from build123d import *

# Parameters (mm, degrees)
SKETCH2_W           = 134.477697302
SKETCH2_H           = 109.076354478
BOSS_EXTRUDE1_DEPTH = 84.074
SKETCH3_R           = 12.7
CUT_EXTRUDE1_DEPTH  = 127
SKETCH4_W           = 81.978128355
SKETCH4_H           = 50.707128689
CUT_EXTRUDE2_DEPTH  = 104.14
BOSS_EXTRUDE2_DEPTH = 25.4
BOSS_EXTRUDE3_DEPTH = 25.4


with BuildPart() as part:
    # Sketch2 → Boss-Extrude1 (new body)
    with BuildSketch(Plane.XY):
        Rectangle(SKETCH2_W, SKETCH2_H)
    extrude(amount=BOSS_EXTRUDE1_DEPTH)

    # Sketch3 → Cut-Extrude1 (cut)
    with BuildSketch(Plane.XY.offset(84.074)):
        Circle(SKETCH3_R)
    extrude(amount=-CUT_EXTRUDE1_DEPTH, mode=Mode.SUBTRACT)

    # Sketch4 → Cut-Extrude2 (cut)
    with BuildSketch(Plane(origin=(0, 54.538177239, 0), x_dir=(1, 0, 0), z_dir=(0, 1, 0))):
        with Locations((-7.023947617, -26.021677284)):
            Rectangle(SKETCH4_W, SKETCH4_H)
    extrude(amount=-CUT_EXTRUDE2_DEPTH, mode=Mode.SUBTRACT)

    # Sketch5 → Boss-Extrude2 (add)
    with BuildSketch(Plane(origin=(67.238848651, 0, 0), x_dir=(0, 0, -1), z_dir=(1, 0, 0))):
        Polygon((-54.326321663, 1.325818935), (-44.711130396, 12.412030691), (-49.504475775, 26.282136468), (-63.913012421, 29.06603049), (-73.528203689, 17.979818734), (-68.734858309, 4.109712956), align=None)
    extrude(amount=BOSS_EXTRUDE2_DEPTH)

    # Sketch6 → Boss-Extrude3 (add)
    with BuildSketch(Plane(origin=(67.238848651, 0, 0), x_dir=(0, 0, -1), z_dir=(1, 0, 0))):
        Polygon((-33.317190853, -32.329584791), (-34.779908073, -16.333922758), (-49.363916354, -9.602842013), (-62.485207415, -18.867423301), (-61.022490195, -34.863085333), (-46.438481914, -41.594166078), align=None)
    extrude(amount=BOSS_EXTRUDE3_DEPTH)


solid = part.part
Geometry: final body of the model. Coordinates: model frame, mm. A direction names the side the tool comes from. Round coordinates to 2 decimals unless told otherwise and drop trailing zeros. Order: outer loops, then holes, each group sorted by start corner. A loop starts at its lowest first (then second) coordinate and runs counter-clockwise, first axis right, second up. Notation, with made-up numbers: (31, -37.75) -> (78, -37.75) arc R15 ccw to (78, -22.75) -> close; hole circle Ø4 at (-34.5, -5.75). An arc over 180 degrees is marked (long way). Put each result on its own line as item: value. Start each with the question number.
Q1. Section A-A on x = 0. Return the cut outline in (y, z), and give its area (3 significant figures).
Q2. Line query: probe 1 along Y at (x, z) = (0, 58.5); probe 2 along Z at (x, y) = (33.5, 22.5); probe 3 along X at (y, z) = (-38, 43.5). Output: solid intervals per line, ascending.
Q3. Reachability of faces 1 (the flat face through (79.761, 23.601, 68.653)), 2 (the flat face through (79.761, -26.753, 61.764)), 3 (the flat face through (79.761, -37.027, 39.97)), 4 (the flat face through (79.761, 19.25, 47.074)), 5 (the flat face through (79.761, 6.791, 49.586)) from +Z, -Z, +X, -X, +Y, -Y: full face, straight path, thin tool, end or side. Return the list, or none.
Q4. Pull-direction query (Y, two-part tool) for faces 6 (the flat face through (-1, 54.538, 60)), 7 (the flat face through (-67.239, -1, 41)), 8 (the flat face through (79.761, 2.737, 61.631)), 9 (the cylindrical face through (-2.75, -12.4, 0.34)); classes: +Y half, -Y half, draft (parallel to the pull), parting line (faces both ways), or undercut.
Q5. Section B-B on y = -5. Return the cut outline in (x, z).
Q6. Section C-C on z = 31. Return the cut outline in (x, y), and give its area (3 significant figures).
Q7. Section D-D on y = -39.5. Return the cut outline in (x, z), and give its area (3 significant figures).
Q8. First-contact query: pin 1 (12 mm diameter, centred on y = -43, z = 35.5, fed in from +X); pin 2 (12 mm diameter, centred on x = 55, y = -25.5, fed in from -Z); pin 3 (12 mm diameter, centred on x = -6.5, z = 23.5, fed in from +Y); pin 4 (4 mm diameter, centred on x = 72.5, y = 26, fed in from +Z). Flat tips, straight axial feed; report the tip coordinate or a pass-through.
Ans:
1. outline: (-54.54, 0) -> (-12.7, 0) -> (-12.7, 0.67) -> (-49.6, 0.67) -> (-49.6, 51.38) -> (-12.7, 51.38) -> (-12.7, 84.07) -> (-54.54, 84.07) -> close; (12.7, 0) -> (54.54, 0) -> (54.54, 0.67) -> (12.7, 0.67) -> close; (12.7, 51.38) -> (54.54, 51.38) -> (54.54, 84.07) -> (12.7, 84.07) -> close
1. area: 3,040 mm2
2. probe 1: y = -54.54 to -12.7, 12.7 to 54.54
2. probe 2: z = 0 to 0.67, 51.38 to 84.07
2. probe 3: x = -67.24 to -48.01, 33.97 to 92.64
3. face 1: +Z, +X, +Y
3. face 2: +Z, +X, -Y
3. face 3: -Z, +X, -Y
3. face 4: -Z, +X, +Y
3. face 5: -Z, +X
4. face 6: +Y half
4. face 7: draft
4. face 8: undercut
4. face 9: undercut
5. outline: (-67.24, 0) -> (-11.67, 0) -> (-11.67, 0.67) -> (-48.01, 0.67) -> (-48.01, 51.38) -> (-11.67, 51.38) -> (-11.67, 84.07) -> (-67.24, 84.07) -> close; (11.67, 0) -> (67.24, 0) -> (67.24, 84.07) -> (11.67, 84.07) -> (11.67, 51.38) -> (33.97, 51.38) -> (33.97, 0.67) -> (11.67, 0.67) -> close
6. outline: (-67.24, -54.54) -> (67.24, -54.54) -> (67.24, 54.54) -> (33.97, 54.54) -> (33.97, -49.6) -> (-48.01, -49.6) -> (-48.01, 54.54) -> (-67.24, 54.54) -> close
6. area: 6,130 mm2
7. outline: (-67.24, 0) -> (67.24, 0) -> (67.24, 43.47) -> (92.64, 43.47) -> (92.64, 50.98) -> (67.24, 50.98) -> (67.24, 84.07) -> (-67.24, 84.07) -> close; hole (-48.01, 0.67) -> (33.97, 0.67) -> (33.97, 51.38) -> (-48.01, 51.38) -> close
7. area: 7,340 mm2
8. pin 1: stops at x = 67.24
8. pin 2: stops at z = 0
8. pin 3: stops at y = -49.6
8. pin 4: stops at z = 68.31
